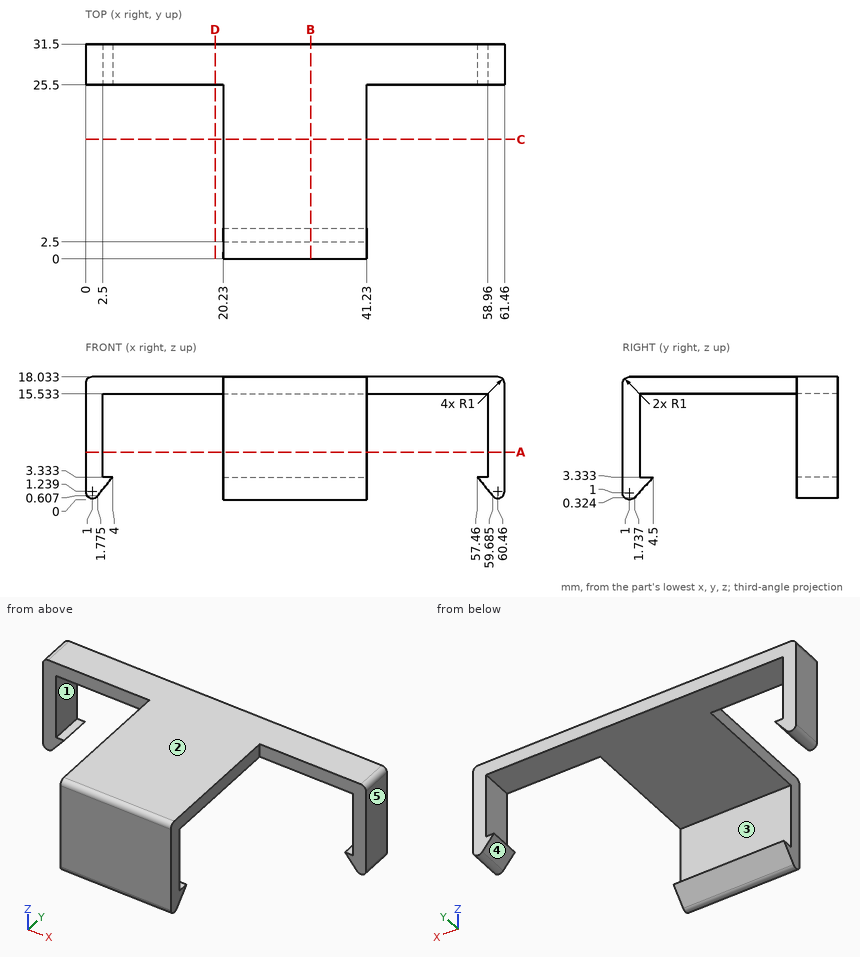
For this review, use the dimensioned drawing (mm, ordinates from the lowest corner) and the shaded views. A direction names the side the tool comes from. Give positions to 0.01 mm unless a question says otherwise; leave off trailing zeros. Loops run counter-clockwise (first coordinate to the right, second up) from the corner with the lowest first, then second, coordinate; pieces in that order, holes last. Notation, with made-up numbers: (32, 39.5) - (81, 39.5) arc R23 ccw to (81, 49.5) - close; hole circle Ø6 at (-24, 29). An arc over 180 degrees is marked (long way). Write each question's results on one line, items separated by ' | '.
(1) For line 1 along X through (y, z) = (28.5, 9.5); line 2 along Z through (x, y) = (15.5, 28); line 3 along Y through (x, z) = (36.5, 10.75), list the stretches that pass through material, from the lowest coordinate up.
Conclusion:
line 1: 0 to 2.5, 58.96 to 61.46 | line 2: 15.53 to 18.03 | line 3: 0 to 2.5
(2) For pin 1 Ø3 at (x, z) = (30, 12) entering from -Y; pin 2 Ø1 at (x, y) = (28.5, 14.5) entering from -Z; pin 3 Ø6 at (y, z) = (20.5, 13.5) entering from -X, all flat-tipped, find the tip position at first contact; note any pin that passes through.
Conclusion:
pin 1: y = 0 | pin 2: z = 15.53 | pin 3: x = 20.23
(3) Take a section at B-B (x = 33). Give the boundary of the cut face in (y, z), then the cut area to 3 significant figures.
Conclusion:
outline: (0, 1) arc R1 ccw to (1.74, 0.32) - (4.5, 3.33) - (2.5, 3.33) - (2.5, 15.53) - (31.5, 15.53) - (31.5, 18.03) - (1, 18.03) arc R1 ccw to (0, 17.03) - close | area: 119 mm^2
(4) For the marked faces 1 and 2, list the 3-axis set-ups (+Z, -Z, +X, -X, +Y, -Y) from which the entire face can be reached by the end or side of a thin tool; tool diameter is ignored.
Conclusion:
face 1: +Y, -Y | face 2: +Z, +X, -X, +Y, -Y
(5) Take a section at C-C (y = 17.5). Give the boundary of the cut face in (x, z), then the cut area to 3 significant figures.
Conclusion:
outline: (20.23, 15.53) - (41.23, 15.53) - (41.23, 18.03) - (20.23, 18.03) - close | area: 52.5 mm^2
(6) Draft analysis for pull direction Z (two halves, no side actions). For the marked faces 3, 4 and 5, state which applies: +Z half, -Z half, draft (parallel to the pull), parting line (faces both ways), or undercut.
Conclusion:
face 3: undercut | face 4: -Z half | face 5: draft
(7) Take a section at D-D (x = 19). Give the boundary of the cut face in (y, z).
Conclusion:
outline: (25.5, 15.53) - (31.5, 15.53) - (31.5, 18.03) - (25.5, 18.03) - close
(8) Take a section at A-A (z = 7). Give the boundary of the cut face in (x, y).
Conclusion:
outline: (0, 25.5) - (2.5, 25.5) - (2.5, 31.5) - (0, 31.5) - close; (20.23, 0) - (41.23, 0) - (41.23, 2.5) - (20.23, 2.5) - close; (58.96, 25.5) - (61.46, 25.5) - (61.46, 31.5) - (58.96, 31.5) - close
